Here's how the part is built. I have some questions about the finished solid (model axes, mm). Face numbers are marked on the shaded views. A direction names the side the tool comes from. Give positions to 0.01 mm unless a question says otherwise; leave off trailing zeros. Order: outer loops, then holes, each group sorted by start corner. A loop starts at its lowest first (then second) coordinate and runs counter-clockwise, first axis right, second up.
from build123d import *

# Parameters (mm, degrees)
F1_DEPTH = 533.4
F2_W     = 1362.075
F2_H     = 679.45
F3_DEPTH = 19.05
F4_W     = 19.05
F4_H     = 660.4
F5_DEPTH = 533.4
F7_D     = 9.525
F7_DEPTH = 9.525
F7_TIP   = 2.8615986981


with BuildPart() as f1:
    # F0 (on Front) → F1 (new body)
    with BuildSketch(Plane.XZ):
        Polygon((-661.9875, 679.45), (-681.0375, 679.45), (-681.0375, 0), (681.0375, 0), (681.0375, 679.45), (661.9875, 679.45), (661.9875, 19.05), (-661.9875, 19.05), align=None)
    extrude(amount=-F1_DEPTH)

    # F2 (on face) → F3 (join)
    with BuildSketch(Plane(origin=(0, 533.4, 0), x_dir=(-1, 0, 0), z_dir=(0, 1, 0))):
        with Locations((0, 339.725)):
            Rectangle(F2_W, F2_H)
    extrude(amount=F3_DEPTH)

    # F4 (on face) → F5 (join, through all)
    with BuildSketch(Plane.XZ):
        with Locations((-342.9, 349.25)):
            Rectangle(F4_W, F4_H)
        with Locations((328.6125, 349.25)):
            Rectangle(F4_W, F4_H)
    extrude(amount=-F5_DEPTH)

    # F7
    with Locations(Plane(origin=(0, 0, 0), x_dir=(1, 0, 0), z_dir=(0, 0, -1))):
        with Locations((-639.1275, -41.91), (-639.1275, -510.54), (639.1275, -41.91), (639.1275, -510.54)):
            Hole(F7_D / 2, depth=F7_DEPTH)
            with Locations((0, 0, -(F7_DEPTH + F7_TIP / 2))):  # 118° drill point
                Cone(0, F7_D / 2, F7_TIP, mode=Mode.SUBTRACT)


solid = f1.part
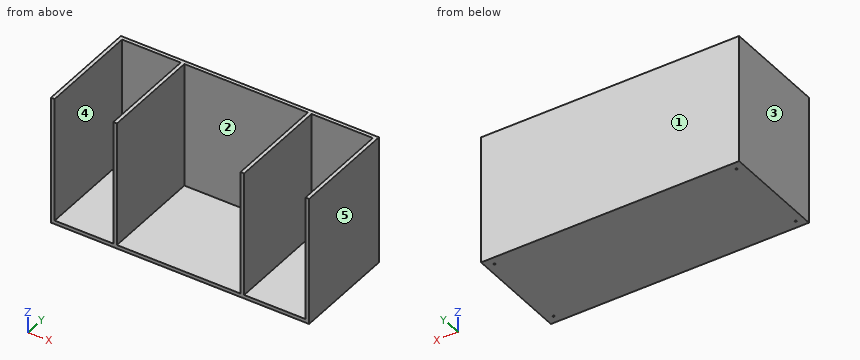
Q1. I'm going to push flat-ended pins straight in: P1, Ø5, axis at x = -223, z = 284.5, coming from the -Y side; P2, Ø15, axis at x = -639.13, y = 41.91, coming from the +Z side. Where does each tip first touch, or does it pass through?
Filled sheet:
P1: stops at y = 533.4
P2: stops at z = 19.05
Q2. Thinking about a two-plate mould opening in X: for the marked faces 1, 2 and 3, which applies, released by +X, released by -X, zero draft, split by the parting line, or undercut?
Filled sheet:
face 1: zero draft
face 2: undercut
face 3: released by -X
Q3. If we section it at B-B on x = 70: List the corners of the cut face in (y, z) for me.
Filled sheet:
outline: (0, 0) - (552.45, 0) - (552.45, 679.45) - (533.4, 679.45) - (533.4, 19.05) - (0, 19.05) - close
Q4. I need wall thicknesses on L1, parallel to X at y = 241.5, z = 133.5 (1 decimal); L2, parallel to X at y = 41.91, z = 5.5 (1 decimal); L3, parallel to Y at x = -609, z = 473. Which ranges of each line are inside material? Lowest first, please.
Filled sheet:
L1: x = -681 to -662, -352.4 to -333.4, 319.1 to 338.1, 662 to 681
L2: x = -681 to -643.9, -634.4 to 634.4, 643.9 to 681
L3: y = 533.4 to 552.45
Q5. For the marked faces 4 and 5, which set-ups out of +Z, -Z, +X, -X, +Y, -Y let a thin tool reach every point of the face, with its end or its side?
Filled sheet:
face 4: +Z, -Y
face 5: +Z, -Z, +X, +Y, -Y
